from build123d import *

# Parameters (mm, degrees)
F1_DEPTH = 15
F3_DEPTH = 10
F4_R     = 0.5
F6_DEPTH = 10


with BuildPart() as f1:
    # F0 (on Right) → F1 (new body)
    with BuildSketch(Plane.YZ):
        with BuildLine():
            Line((4.2912878475, 5), (-4.2912878475, 5))
            ThreePointArc((-4.2912878475, 5), (-7.5, 0), (-4.2912878475, -5))
            Line((-4.2912878475, -5), (4.2912878475, -5))
            ThreePointArc((4.2912878475, -5), (7.5, 0), (4.2912878475, 5))
        make_face()
    extrude(amount=F1_DEPTH)

    # F2 (on face) → F3 (join)
    with BuildSketch(Plane.YZ.offset(15)):
        with BuildLine():
            Line((-4.2912878475, 5), (-7.5, 5))
            Line((-7.5, 5), (-7.5, 0))
            ThreePointArc((-7.5, 0), (-6.628827236, 2.9705148408), (-4.2912878475, 5))
        make_face()
        with BuildLine():
            Line((7.5, 5), (4.2912878475, 5))
            ThreePointArc((4.2912878475, 5), (6.628827236, 2.9705148408), (7.5, 0))
            Line((7.5, 0), (7.5, 5))
        make_face()
        with BuildLine():
            Line((4.2912878475, 5), (-4.2912878475, 5))
            ThreePointArc((-4.2912878475, 5), (-6.628827236, 2.9705148408), (-7.5, 0))
            ThreePointArc((-7.5, 0), (-6.628827236, -2.9705148408), (-4.2912878475, -5))
            Line((-4.2912878475, -5), (4.2912878475, -5))
            ThreePointArc((4.2912878475, -5), (6.628827236, -2.9705148408), (7.5, 0))
            ThreePointArc((7.5, 0), (6.628827236, 2.9705148408), (4.2912878475, 5))
        make_face()
        with BuildLine():
            ThreePointArc((-4.2912878475, -5), (-6.628827236, -2.9705148408), (-7.5, 0))
            Line((-7.5, 0), (-7.5, -5))
            Line((-7.5, -5), (-4.2912878475, -5))
        make_face()
        with BuildLine():
            Line((7.5, -5), (7.5, 0))
            ThreePointArc((7.5, 0), (6.628827236, -2.9705148408), (4.2912878475, -5))
            Line((4.2912878475, -5), (7.5, -5))
        make_face()
    extrude(amount=F3_DEPTH)

    # F4
    f4_edges = [f1.edges().sort_by_distance(p)[0] for p in [
        (20, -7.5, 5),
        (20, 7.5, 5),
        (20, -7.5, -5),
        (20, 7.5, -5),
    ]]
    fillet(f4_edges, radius=F4_R)

    # F5 (on face) → F6 (join)
    with BuildSketch(Plane.YZ.offset(25)):
        with BuildLine():
            Line((1.1180339887, 1), (-1.1180339887, 1))
            ThreePointArc((-1.1180339887, 1), (0, -1.5), (1.1180339887, 1))
        make_face()
    extrude(amount=F6_DEPTH)


solid = f1.part
Read the model definition and answer for the solid it produces. Units are mm, in the model's axes. A direction names the side the tool comes from. Give positions to 0.01 mm unless a question says otherwise; leave off trailing zeros. Loops run counter-clockwise (first coordinate to the right, second up) from the corner with the lowest first, then second, coordinate; pieces in that order, holes last. Notation, with made-up numbers: (11.5, -5.5) - (27.5, -5.5) arc R7 cw to (27.5, -0.5) - close; hole circle Ø2 at (-1.5, 46.5). An arc over 180 degrees is marked (long way). Answer as CSV lines item,"result". Start each with the question number.
1) Which of the six approach directions +Z, -Z, +X, -X, +Y, -Y give full straight-line access (tool end or side, diameter ignored) to faces 1 (the face through (7.4, -7.5, 0.1)), 2 (the face through (15, 7, -4)), 3 (the face through (15, 7, 4)), 4 (the face through (15, -7, 4))?
2) Straight lines are drawn through the part: L1, parallel to X at y = -3, z = 0; L2, parallel to X at y = 5.25, z = 4.5; L3, parallel to Y at x = 10, z = 4. For each, find the intervals that lie inside material, in ascending order. Write a range as from..to.
3) Find section D-D (z = -0.75). Write down the section's boundary in (x, y), then the cut area to 3 significant figures.
4) Find section C-C (x = 4). Write down the section's boundary in (y, z).
5) Find section B-B (z = -3.25). Write down the section's boundary in (x, y), then the cut area to 3 significant figures.
6) Each of these flat-tipped pins is pushed along its axis until it touches: pin 1 Ø2.5 at (x, y) = (32.5, 0) entering from +Z; pin 2 Ø4 at (y, z) = (5, 1.5) entering from +X; pin 3 Ø1 at (x, z) = (26.5, -0.5) entering from -Y. Where does it stop, or does it pass through?
7) Find section A-A (y = 0). Write down the section's boundary in (x, z).
Findings below:
1,face 1,"-X, -Y"
1,face 2,"-Z, -X, +Y"
1,face 3,"+Z, -X, +Y"
1,face 4,"+Z, -X, -Y"
2,L1,"0..25"
2,L2,"15..25"
2,L3,"-5.77..5.77"
3,outline,"(0, -7.45) - (15, -7.45) - (15, -7.5) - (25, -7.5) - (25, -1.3) - (35, -1.3) - (35, 1.3) - (25, 1.3) - (25, 7.5) - (15, 7.5) - (15, 7.45) - (0, 7.45) - close"
3,area,"399 mm^2"
4,outline,"(-4.29, -5) - (4.29, -5) arc R5.5 ccw to (4.29, 5) - (-4.29, 5) arc R5.5 ccw to start"
5,outline,"(0, -6.44) - (15, -6.44) - (15, -7.5) - (25, -7.5) - (25, 7.5) - (15, 7.5) - (15, 6.44) - (0, 6.44) - close"
5,area,"343 mm^2"
6,pin 1,"z = 1"
6,pin 2,"x = 25"
6,pin 3,"y = -1.5"
7,outline,"(0, -5) - (25, -5) - (25, -1.5) - (35, -1.5) - (35, 1) - (25, 1) - (25, 5) - (0, 5) - close"
